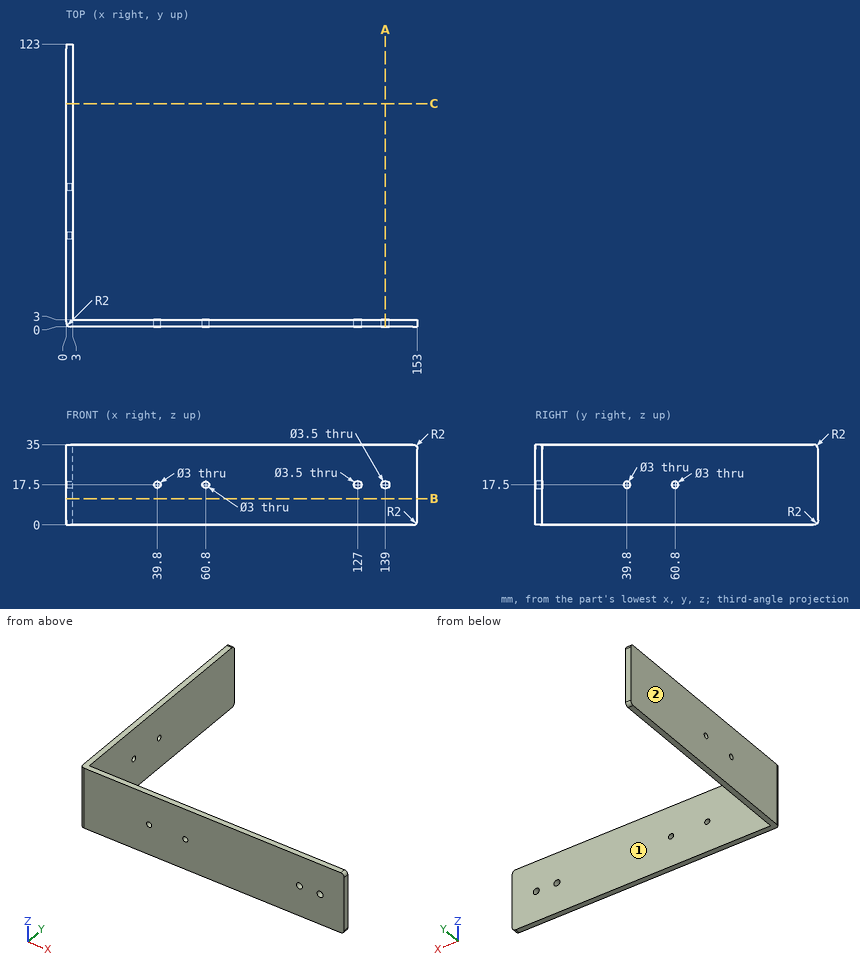
Study the drawing (mm; zero at the part's minimum x, y, z) and answer. A direction names the side the tool comes from. Give positions to 0.01 mm unless a question says otherwise; leave off trailing zeros. Write each loop counter-clockwise with the first axis right and the second up, starting at its lowest first coordinate (ties: lowest second). Pieces come first, ordered by that corner, then holes. Notation, with made-up numbers: (26, 2) -> (32, 2) arc R11 ccw to (32, 13) -> close; hole circle Ø3 at (43, 85.25). An arc over 180 degrees is marked (long way). Answer as a JSON object with one key per item and string values. Group by question number.
1) Consider L1, parallel to Z at x = 127, y = 1; L2, parallel to X at y = 2.35, z = 17.5; L3, parallel to Y at x = 1.55, z = 17.5. Determine where each line is inside the solid, lowest interval first. Write a range as from..to.
2) Find section A-A (x = 139). Write down the section's boundary in (y, z), and give its area (3 significant figures).
3) Find section B-B (z = 11.5). Write down the section's boundary in (x, y), and give its area (3 significant figures).
4) Each of these flat-tipped pins is pushed along its axis until it touches: P1, Ø5, axis at x = 39.8, z = 17.5, coming from the +Y side; P2, Ø2.5, axis at y = 60.8, z = 17.5, coming from the -X side; P3, Ø1.5, axis at y = 102.5, z = 5, coming from the +X side. Where does it stop, or does it pass through?
5) A tool of negligible diameter and unlimited length cuts with its end or side. For the marked faces 1 and 2, from which of +Z, -Z, +X, -X, +Y, -Y can it reach the whole face along a straight path? Write none if from no direction.
6) Find section C-C (y = 97). Write down the section's boundary in (x, z), and give its area (3 significant figures).
Values follow:
{
 "1": {"L1": "z = 0..15.75, 19.25..35", "L2": "x = 0..38.3, 41.3..59.3, 62.3..125.25, 128.75..137.25, 140.75..153", "L3": "y = 0.05..38.3, 41.3..59.3, 62.3..123"},
 "2": {"outline": "(0, 0) -> (3, 0) -> (3, 15.75) -> (0, 15.75) -> close; (0, 19.25) -> (3, 19.25) -> (3, 35) -> (0, 35) -> close", "area": "94.5 mm2"},
 "3": {"outline": "(0, 2) arc R2 ccw to (2, 0) -> (153, 0) -> (153, 3) -> (3, 3) -> (3, 123) -> (0, 123) -> close", "area": "818 mm2"},
 "4": {"P1": "stops at y = 3", "P2": "passes through", "P3": "stops at x = 3"},
 "5": {"face 1": "+Z, -Z, +X, +Y", "face 2": "+Z, -Z, -X, +Y, -Y"},
 "6": {"outline": "(0, 0) -> (3, 0) -> (3, 35) -> (0, 35) -> close", "area": "105 mm2"}
}
